Here's how the part is built. I have some questions about the finished solid (model axes, mm). A direction names the side the tool comes from. Coordinates: 2 decimals unless noted, no trailing zeros. Order: outer loops, then holes, each group sorted by start corner. A loop starts at its lowest first (then second) coordinate and runs counter-clockwise, first axis right, second up. Notation, with made-up numbers: (-4.5, 85.5) - (50.5, 85.5) arc R20 cw to (50.5, 122.5) - close; hole circle Ø10 at (12.5, -4). An arc over 180 degrees is marked (long way). Use CSV: the item, a comma, the result in double quotes. Start each with the question number.
from build123d import *

# Parameters (mm, degrees)
SKETCH_1_R           = 30
EXTRUDE_1_DEPTH      = 15
SKETCH_2_OUTSIDE_W   = 79.234
SKETCH_2_OUTSIDE_H   = 79.234
SKETCH_2_OUTSIDE_R   = 27.5
CUT_EXTRUDE_1_DEPTH  = 3.8
SKETCH_2_3_OUTSIDE_W = 79.234
SKETCH_2_3_OUTSIDE_H = 79.234
SKETCH_2_3_OUTSIDE_R = 26.5
CUT_EXTRUDE_2_DEPTH  = 3.3
SKETCH_4_R           = 2.175
EXTRUDE_2_DEPTH      = 36
CHAMFER_1_SIZE       = 0.5
FILLET_1_R           = 1
FILLET_2_R           = 0.4


with BuildPart() as part:
    # Sketch 1 → Extrude 1 (new body)
    with BuildSketch(Plane(origin=(0, 0, 0), x_dir=(1, 0, 0), z_dir=(0, 1, 0))):
        Circle(SKETCH_1_R)
    extrude(amount=EXTRUDE_1_DEPTH)

    # Sketch 2 outside → Cut-Extrude 1 (cut)
    with BuildSketch(Plane(origin=(0, 0, 0), x_dir=(1, 0, 0), z_dir=(0, 1, 0))):
        Rectangle(SKETCH_2_OUTSIDE_W, SKETCH_2_OUTSIDE_H)
        Circle(SKETCH_2_OUTSIDE_R, mode=Mode.SUBTRACT)
    extrude(amount=CUT_EXTRUDE_1_DEPTH, mode=Mode.SUBTRACT)

    # Sketch 2_3 outside → Cut-Extrude 2 (cut)
    with BuildSketch(Plane(origin=(0, 0, 0), x_dir=(1, 0, 0), z_dir=(0, 1, 0))):
        Rectangle(SKETCH_2_3_OUTSIDE_W, SKETCH_2_3_OUTSIDE_H)
        Circle(SKETCH_2_3_OUTSIDE_R, mode=Mode.SUBTRACT)
    extrude(amount=CUT_EXTRUDE_2_DEPTH, mode=Mode.SUBTRACT)

    # Sketch 3 → Cut-Revolve 1 (revolve, cut)
    with BuildSketch(Plane.XY):
        with BuildLine():
            Line((-42.194966184, 4.5), (-30, 4.5))
            ThreePointArc((-30, 4.5), (-27.555432596, 6.326286214), (-25, 7.993917882))
            ThreePointArc((-25, 7.993917882), (-24.402555654, 8.351420449), (-23.8, 8.700239193))
            ThreePointArc((-23.8, 8.700239193), (-12.309823173, 13.398399257), (0, 15))
            Line((0, 15), (0, 24.071462315))
            Line((0, 24.071462315), (-42.194966184, 24.071462315))
            Line((-42.194966184, 24.071462315), (-42.194966184, 4.5))
        make_face()
        with BuildLine():
            ThreePointArc((-23.8, 8.700239193), (-24.402555654, 8.351420449), (-25, 7.993917882))
            Line((-25, 7.993917882), (-24, 7.993917882))
            Line((-24, 7.993917882), (-24, 6.993917882))
            Line((-24, 6.993917882), (-23.8, 6.993917882))
            Line((-23.8, 6.993917882), (-23.8, 8.700239193))
        make_face()
    revolve(axis=Axis((0, 0, 0), (0, 1, 0)), mode=Mode.SUBTRACT)

    # Sketch 4 → Extrude 2 (add)
    with BuildSketch(Plane(origin=(0, 0, 0), x_dir=(0, 0, -1), z_dir=(1, 0, 0))):
        with Locations((0, 4.5)):
            Circle(SKETCH_4_R)
    extrude(amount=EXTRUDE_2_DEPTH)

    # Chamfer 1
    chamfer_1_edges = [part.edges().sort_by_distance(p)[0] for p in [
        (-26.5, 0, 0),
    ]]
    chamfer(chamfer_1_edges, length=CHAMFER_1_SIZE)

    # Fillet 1
    fillet_1_edges = [part.edges().sort_by_distance(p)[0] for p in [
        (25, 7.993917882, 0),
        (23.8, 8.700239193, 0),
    ]]
    fillet(fillet_1_edges, radius=FILLET_1_R)

    # Fillet 2
    fillet_2_edges = [part.edges().sort_by_distance(p)[0] for p in [
        (24, 7.993917882, 0),
    ]]
    fillet(fillet_2_edges, radius=FILLET_2_R)


solid = part.part
Item 1: Please list where these lines run through material, in increasing order: line 1 along Z through (x, y) = (0, 7.2); line 2 along Z through (x, y) = (0, 7.3); line 3 along X through (y, z) = (7.75, 14). Write a range as from..to.
Item 2: For pin 1 Ø8 at (y, z) = (9, -9) entering from +X; pin 2 Ø3 at (x, z) = (5, -14.5) entering from +Y; pin 3 Ø1 at (y, z) = (10.5, 8) entering from +X, each with a flat end and sliding along its axis, tell me the tip position at first contact or that it passes through.
Item 3: For faces 1 (the cylindrical face through (32.214, 2.377, 0.471)), 2 (the cylindrical face through (14.246, 1.88, -22.345)), 3 (the flat face through (-1.7, 7.994, -24.5)), which set-ups out of +Z, -Z, +X, -X, +Y, -Y let a thin tool reach every point of the face, with its end or its side?
Item 4: Suppose I cut it at A-A on y = 13.5. Write out the boundary of the cut face in (x, z), then the cut area to 3 significant figures.
Item 5: We'd pull the mould along X, two halves only. Please class faces 4 (the flat face through (-25, 3.3, -10)), 5 (the cylindrical face through (23.977, 7.29, 1.055)), 6 (the flat face through (36, 5, 0)), 7 (the cylindrical face through (18.89, 7.56, -14.48)): released by +X, released by -X, zero draft, split by the parting line, or undercut.
Item 6: Suppose I cut it at B-B on y = 10. Write out the boundary of the cut face in (x, z).
Item 7: Suppose I cut it at C-C on y = 5.75. Write out the boundary of the cut face in (x, z).
Here are the results:
1,line 1,"-26.26..-24, -23.8..23.8, 24..26.26"
1,line 2,"-26.11..-24, -23.8..23.8, 24..26.11"
1,line 3,"-21.19..-19.53, -19.25..19.25, 19.53..21.19"
2,pin 1,"x = 28.08"
2,pin 2,"y = 12.97"
2,pin 3,"x = 19.82"
3,face 1,"+X"
3,face 2,"-Y"
3,face 3,"+Y"
4,outline,"circle Ø23.84 at (0, 0)"
4,area,"446 mm^2"
5,face 4,"zero draft"
5,face 5,"undercut"
5,face 6,"released by +X"
5,face 7,"undercut"
6,outline,"circle Ø42.71 at (0, 0)"
7,outline,"(28.31, -1.78) - (36, -1.78) - (36, 1.78) - (28.31, 1.78) arc R28.36 ccw (long way) to start"
